For this review, take the finished solid that the model builds, in its own axes (mm). A direction names the side the tool comes from. Coordinates: 2 decimals unless noted, no trailing zeros. Order: outer loops, then holes, each group sorted by start corner. A loop starts at its lowest first (then second) coordinate and runs counter-clockwise, first axis right, second up. Notation, with made-up numbers: (7.5, 61.5) -> (59.5, 61.5) arc R23 ccw to (59.5, 81.5) -> close; hole circle Ø8 at (-12, 36). An arc over 180 degrees is marked (long way). Return JSON: item names as keys, results as strings. Group by question number.
Item 1: Draft analysis for pull direction Z (two halves, no side actions). For faces 3 (the flat face through (493, 13, 25.75)), 4 (the flat face through (493, 11, 0)), 5 (the flat face through (0, 1, 15)), 6 (the flat face through (493, 25.6, 16)), state which applies: +Z half, -Z half, draft (parallel to the pull), parting line (faces both ways), or undercut.
Item 2: Take a section at B-B (z = 17). Write out the cut boundary in (x, y).
Item 3: Insertion check: pin 1 (0.6 mm diameter, centred on x = 336, z = 6.5, fed in from -Y); pin 2 (0.5 mm diameter, centred on x = 354, z = 1, fed in from +Y); pin 3 (1.5 mm diameter, centred on x = 251, y = 26, fed in from -Z); pin 4 (2 mm diameter, centred on y = 3.5, z = 9, fed in from -X). Each pin has a flat end and moves straight along its axis. Give the tip position at first contact, or say it passes through.
Item 4: Take a section at C-C (x = 277). Write out the cut boundary in (y, z), then the cut area to 3 significant figures.
Item 5: For line 1 along Z through (x, y) = (423.5, 15.25); line 2 along Y through (x, z) = (473, 22.75); line 3 along Y through (x, z) = (619, 6.5), list the stretches that pass through material, from the lowest coordinate up.
Item 6: Take a section at A-A (y = 12.5). Write out the cut boundary in (x, z).
Item 7: Machinability: for faces 1 (the flat face through (493, 27.2, 16)), 2 (the flat face through (493, 1.6, 14)), which of the approach directions +Z, -Z, +X, -X, +Y, -Y give a long, thin tool a straight path to every point of the face, cutting with its end or side? Answer none if there is none.
```python
from build123d import *

# Parameters (mm, degrees)
F1_DEPTH = 1000


with BuildPart() as f1:
    # F0 (on Right) → F1 (new body)
    with BuildSketch(Plane.YZ):
        with BuildLine():
            Line((27.2, 5.35), (27.2, 27.35))
            Line((27.2, 27.35), (0, 27.35))
            Line((0, 27.35), (0, 0))
            Line((0, 0), (22, 0))
            Line((22, 0), (22, 1.6))
            ThreePointArc((22, 1.6), (21.926777, 1.776777), (21.75, 1.85))
            Line((21.75, 1.85), (21.37081, 1.85))
            ThreePointArc((21.37081, 1.85), (21.147203, 1.781662), (21, 1.6))
            Line((21, 1.6), (1.6, 1.6))
            Line((1.6, 1.6), (1.6, 13.675))
            Line((1.6, 13.675), (1.6, 25.75))
            Line((1.6, 25.75), (25.6, 25.75))
            Line((25.6, 25.75), (25.6, 6.95))
            Line((25.6, 6.95), (24.7, 6.95))
            ThreePointArc((24.7, 6.95), (24.552797, 7.131662), (24.32919, 7.2))
            Line((24.32919, 7.2), (23.85, 7.2))
            ThreePointArc((23.85, 7.2), (23.673223, 7.126777), (23.6, 6.95))
            Line((23.6, 6.95), (23.6, 5.85))
            ThreePointArc((23.6, 5.85), (23.746447, 5.496447), (24.1, 5.35))
            Line((24.1, 5.35), (27.2, 5.35))
        make_face()
    extrude(amount=F1_DEPTH)


solid = f1.part
```
Findings below:
{
 "1": {"face 3": "undercut", "face 4": "-Z half", "face 5": "draft", "face 6": "undercut"},
 "2": {"outline": "(0, 0) -> (1000, 0) -> (1000, 1.6) -> (0, 1.6) -> close; (0, 25.6) -> (1000, 25.6) -> (1000, 27.2) -> (0, 27.2) -> close"},
 "3": {"pin 1": "stops at y = 0", "pin 2": "stops at y = 22", "pin 3": "stops at z = 5.35", "pin 4": "passes through"},
 "4": {"outline": "(0, 0) -> (22, 0) -> (22, 1.6) arc R0.25 ccw to (21.75, 1.85) -> (21.37, 1.85) arc R0.4 ccw to (21, 1.6) -> (1.6, 1.6) -> (1.6, 25.75) -> (25.6, 25.75) -> (25.6, 6.95) -> (24.7, 6.95) arc R0.4 ccw to (24.33, 7.2) -> (23.85, 7.2) arc R0.25 ccw to (23.6, 6.95) -> (23.6, 5.85) arc R0.5 ccw to (24.1, 5.35) -> (27.2, 5.35) -> (27.2, 27.35) -> (0, 27.35) -> close", "area": "154 mm2"},
 "5": {"line 1": "z = 0 to 1.6, 25.75 to 27.35", "line 2": "y = 0 to 1.6, 25.6 to 27.2", "line 3": "y = 0 to 1.6, 23.6 to 27.2"},
 "6": {"outline": "(0, 0) -> (1000, 0) -> (1000, 1.6) -> (0, 1.6) -> close; (0, 25.75) -> (1000, 25.75) -> (1000, 27.35) -> (0, 27.35) -> close"},
 "7": {"face 1": "+Z, -Z, +X, -X, +Y", "face 2": "+X, -X"}
}
